from build123d import *

# Parameters (mm, degrees)
F0_W     = 500
F0_H     = 500
F0_R     = 15
F0_R_2   = 12.05
F1_DEPTH = 30
F2_R     = 5
F3_R     = 200
F4_DEPTH = 5


with BuildPart() as f1:
    # F0 (on Top) → F1 (new body)
    with BuildSketch(Plane.XY):
        Rectangle(F0_W, F0_H)
        with Locations((-200, -200)):
            Circle(F0_R, mode=Mode.SUBTRACT)
        with Locations((200, -200)):
            Circle(F0_R, mode=Mode.SUBTRACT)
        with Locations((27.5, -47.631397)):
            Circle(F0_R_2, mode=Mode.SUBTRACT)
        with Locations((82.5, -47.631397)):
            Circle(F0_R_2, mode=Mode.SUBTRACT)
        with Locations((137.5, -47.631397)):
            Circle(F0_R_2, mode=Mode.SUBTRACT)
        with Locations((-200, 200)):
            Circle(F0_R, mode=Mode.SUBTRACT)
        Circle(F0_R_2, mode=Mode.SUBTRACT)
        with Locations((55, 0)):
            Circle(F0_R_2, mode=Mode.SUBTRACT)
        with Locations((110, 0)):
            Circle(F0_R_2, mode=Mode.SUBTRACT)
        with Locations((165, 0)):
            Circle(F0_R_2, mode=Mode.SUBTRACT)
        with Locations((200, 200)):
            Circle(F0_R, mode=Mode.SUBTRACT)
    extrude(amount=F1_DEPTH)

    # F2
    f2_edges = [f1.edges().sort_by_distance(p)[0] for p in [
        (-250, -250, 15),
        (250, -250, 15),
        (250, 250, 15),
        (-250, 250, 15),
    ]]
    fillet(f2_edges, radius=F2_R)

    # F3 (on face) → F4 (cut)
    with BuildSketch(Plane.XY.offset(30)):
        Circle(F3_R)
    extrude(amount=-F4_DEPTH, mode=Mode.SUBTRACT)


solid = f1.part
Work out the finished part from the listing and answer in its coordinate system (mm). A direction names the side the tool comes from. Give positions to 0.01 mm unless a question says otherwise; leave off trailing zeros. Order: outer loops, then holes, each group sorted by start corner. A loop starts at its lowest first (then second) coordinate and runs counter-clockwise, first axis right, second up. Notation, with made-up numbers: (35.5, 35.25) -> (94.5, 35.25) arc R7 cw to (94.5, 42.25) -> close; hole circle Ø7 at (-26, 88.5). An arc over 180 degrees is marked (long way). One line per item, written item: value.
Item 1: Straight lines are drawn through the part: probe 1 along Y at (x, z) = (-200, 18.75); probe 2 along X at (y, z) = (0, 6.25); probe 3 along Y at (x, z) = (165, 9.25). For each, find the intervals that lie inside material, in ascending order.
Answer sheet:
probe 1: -250 to -215, -185 to 185, 215 to 250
probe 2: -250 to -12.05, 12.05 to 42.95, 67.05 to 97.95, 122.05 to 152.95, 177.05 to 250
probe 3: -250 to -12.05, 12.05 to 250
Item 2: Find section A-A, the plane y = -209. Give the vertices of the cut face in (x, z).
Answer sheet:
outline: (-250, 0) -> (-212, 0) -> (-212, 30) -> (-250, 30) -> close; (-188, 0) -> (188, 0) -> (188, 30) -> (-188, 30) -> close; (212, 0) -> (250, 0) -> (250, 30) -> (212, 30) -> close
Item 3: Find section C-C, the plane y = 0. Give the vertices of the cut face in (x, z).
Answer sheet:
outline: (-250, 0) -> (-12.05, 0) -> (-12.05, 25) -> (-200, 25) -> (-200, 30) -> (-250, 30) -> close; (12.05, 0) -> (42.95, 0) -> (42.95, 25) -> (12.05, 25) -> close; (67.05, 0) -> (97.95, 0) -> (97.95, 25) -> (67.05, 25) -> close; (122.05, 0) -> (152.95, 0) -> (152.95, 25) -> (122.05, 25) -> close; (177.05, 0) -> (250, 0) -> (250, 30) -> (200, 30) -> (200, 25) -> (177.05, 25) -> close
Item 4: Determine the mould class of faces 3 (the flat face through (-3, -250, 15)), 4 (the cylindrical face through (190.764, 60.075, 27.535)), 5 (the cylindrical face through (24.888, -59.395, 12.325)), 6 (the flat face through (250, -3, 15)) for opening direction X: released by +X, released by -X, zero draft, split by the parting line, or undercut.
Answer sheet:
face 3: zero draft
face 4: undercut
face 5: undercut
face 6: released by +X
Item 5: A tool of negligible diameter and unlimited length cuts with its end or side. For faces 1 (the flat face through (-3, -42, 25)), 2 (the flat face through (-3, 250, 15)), from which of +Z, -Z, +X, -X, +Y, -Y can it reach the whole face along a straight path? Write none if from no direction.
Answer sheet:
face 1: +Z
face 2: +Z, -Z, +X, -X, +Y
Item 6: Find section B-B, the plane x = 0. Give the vertices of the cut face in (y, z).
Answer sheet:
outline: (-250, 0) -> (-12.05, 0) -> (-12.05, 25) -> (-200, 25) -> (-200, 30) -> (-250, 30) -> close; (12.05, 0) -> (250, 0) -> (250, 30) -> (200, 30) -> (200, 25) -> (12.05, 25) -> close
Item 7: Find section D-D, the plane z = 16.75. State how many separate pieces and enclosed holes the cut face has, plus the area to 3 significant figures.
Answer sheet:
separate pieces: 1
enclosed holes: 11
area: 244,000 mm²
Item 8: A flat-ended cylindrical pin translates along its axis: P1, Ø21.5, axis at x = 55, y = 0, coming from the -Z side. Find the tip coordinate at first contact, or state that the pin passes through.
Answer sheet:
P1: through
